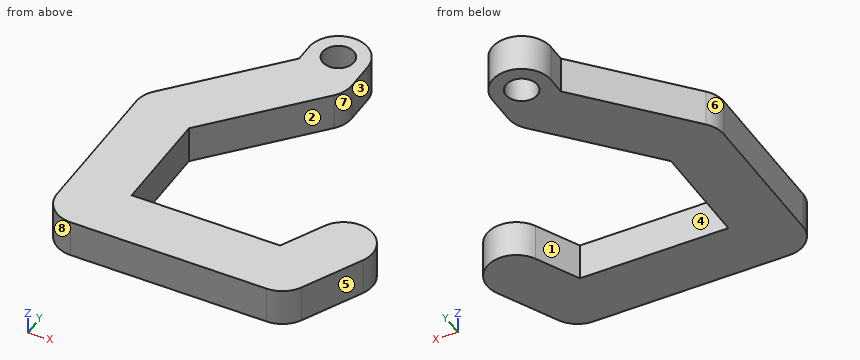
Autodesk Inventor part; units mm, degrees
ref_plane "YZ Plane" through (0, 0, 0) normal (1, 0, 0) x (0, 1, 0)
ref_plane "XZ Plane" through (0, 0, 0) normal (0, 1, 0) x (-1, 0, 0)
ref_plane "XY Plane" through (0, 0, 0) normal (0, 0, 1) x (1, 0, 0)
sketch "Sketch1" plane through (0, 0, 0) normal (0, 0, 1) x (1, 0, 0)
  circle A0 centre (0, 0) radius 1.6
  arc A1 (3, 0) -> (-3, 0) centre (0, 0) ccw
  line L0 (-3, 0) -> (-3, -1.8541)
  line L1 (-3, -3) -> (3, -3) construction
  line L2 (3, -3) -> (3, 0)
  arc A2 (-2.2361, -1) -> (-3, -3) centre (0, -3) ccw construction
  arc A3 (-13, -29.1803) -> (-10, -32.1803) centre (-10, -29.1803) ccw
  arc A4 (7, -29.1803) -> (12.6833, -30.522) centre (10, -29.1803) ccw
  arc A5 (15.6833, -24.522) -> (10.3167, -21.8387) centre (13, -23.1803) ccw
  arc A6 (-12.2361, -12.1803) -> (-13, -14.1803) centre (-10, -14.1803) ccw
  line L3 (-10, -29.1803) -> (10, -29.1803) construction
  line L4 (-7.7639, -16.1803) -> (-7, -15.3262)
  line L5 (-12.2361, -12.1803) -> (-3, -1.8541)
  line L6 (-13, -14.1803) -> (-13, -29.1803)
  line L7 (-7, -14.1803) -> (-7, -15.3262)
  line L8 (-10, -26.1803) -> (-7, -26.1803)
  line L9 (-10, -32.1803) -> (10, -32.1803)
  line L10 (10.3167, -21.8387) -> (7.3167, -27.8387)
  line L11 (12.6833, -30.522) -> (15.6833, -24.522)
  line L12 (-3, -1.8541) -> (-2.2361, -1) construction
  arc A7 (3, -3) -> (-2.2361, -1) centre (0, -3) ccw
  arc A8 (-3, -3) -> (2.2361, -5) centre (0, -3) ccw construction
  line L13 (-3, -1.8541) -> (-3, -3) construction
  arc A9 (2.2361, -5) -> (3, -3) centre (0, -3) ccw
  line L14 (-7, -15.3262) -> (2.2361, -5)
  line L15 (-7, -15.3262) -> (-7, -26.1803)
  arc A10 (-13, -14.1803) -> (-7, -14.1803) centre (-10, -14.1803) ccw construction
  line L16 (-7, -26.1803) -> (10, -26.1803)
  line L17 (-7, -26.1803) -> (-7, -29.1803)
  arc A11 (-10, -26.1803) -> (-13, -29.1803) centre (-10, -29.1803) ccw construction
  arc A12 (-10, -32.1803) -> (-10, -26.1803) centre (-10, -29.1803) ccw construction
  arc A13 (7.3167, -27.8387) -> (7, -29.1803) centre (10, -29.1803) ccw construction
  arc A14 (10, -26.1803) -> (7.3167, -27.8387) centre (10, -29.1803) ccw construction
  arc A15 (12.6833, -30.522) -> (10, -26.1803) centre (10, -29.1803) ccw construction
  arc A16 (10.3167, -21.8387) -> (15.6833, -24.522) centre (13, -23.1803) ccw construction
  point P0 (0, -29.1803)
  point P1 (8.1459, -26.1803)
  dimension "d0" = 3.2
  dimension "d1" = 6
  dimension "d2" = 3
  dimension "d3" = 6
  dimension "d4" = 6
  dimension "d5" = 6
  dimension "d6" = 6
  dimension "d7" = 15
  dimension "d8" = 6
  dimension "d9" = 15
  dimension "d10" = 20
  dimension "d11" = 3
  dimension "d12" = 6
extrude "Extrusion1" add sketch "Sketch1" along normal blind 3.8
properties part number "carlig 2"
Build history of the part. All positions in model axes, mm. Face numbers are marked on the shaded views. A direction names the side the tool comes from. Round coordinates to 2 decimals unless told otherwise and drop trailing zeros. Write each loop counter-clockwise with the first axis right and the second up, starting at its lowest first coordinate (ties: lowest second). Pieces come first, ordered by that corner, then holes. Notation, with made-up numbers: M -27,41.5 L 2,41.5 A18 cw 2,64.5 Z; hole C 73,53.25 d8. An arc over 180 degrees is marked long. Answer as a JSON object with one key per item and string values. Group by question number.
(1) Cut at A-A (z = 2.3). Give the cut face in (x, y).
(2) Cut at D-D (y = -17). Give the cut face in (x, z).
(3) Drill centre lines: L1, parallel to Y at x = 0, z = 1.2; L2, parallel to Y at x = -0.25, z = 2.1; L3, parallel to Y at x = 3.75, z = 2.85. Where is each one in solid material? Low to high.
(4) Flat gauge pins, fed straight in: pin 1 (2 mm diameter, centred on x = 0, y = -1, fed in from +Z); pin 2 (1.1 mm diameter, centred on y = -19.5, z = 1, fed in from +X); pin 3 (1.5 mm diameter, centred on y = -2, z = 1.5, fed in from +X); pin 4 (1.5 mm diameter, centred on y = -1, z = 1.5, fed in from -X). Where does each tip first touch, or does it go through?
(5) Mould opens along Y. For the marked faces 6, 7 and 8 say: pulls with the +Y half, pulls with the -Y half, needs draft (parallel to the pull), parting line crosses it, or undercut.
(6) Cut at C-C (y = -23.5). Give the cut face in (x, z), and give its area (3 significant figures).
(7) Cut at B-B (x = 0). Give the cut face in (y, z).
(8) Which spindle directions (+Z, -Z, +X, -X, +Y, -Y) get a long thin tool onto all of the face, cutting with end or side? Do the marked faces 1, 2, 3, 4 and 5. Say none if no direction does.
Responses:
{
 "1": {"outline": "M -13,-29.18 A3 ccw -10,-32.18 L 10,-32.18 A3 ccw 12.68,-30.52 L 15.68,-24.52 A3 ccw 10.32,-21.84 L 8.15,-26.18 L -7,-26.18 L -7,-15.33 L 2.24,-5 A3 ccw 3,-3 L 3,0 A3 ccw -3,0 L -3,-1.85 L -12.24,-12.18 A3 ccw -13,-14.18 Z; hole C 0,0 d3.2"},
 "2": {"outline": "M -13,0 L -7,0 L -7,3.8 L -13,3.8 Z"},
 "3": {"L1": "y = -32.18 to -26.18, -7.5 to -1.6, 1.6 to 3", "L2": "y = -32.18 to -26.18, -7.78 to -1.58, 1.58 to 2.99", "L3": "y = -32.18 to -26.18"},
 "4": {"pin 1": "stops at z = 3.8", "pin 2": "stops at x = -7", "pin 3": "stops at x = 3", "pin 4": "stops at x = -3"},
 "5": {"face 6": "pulls with the +Y half", "face 7": "undercut", "face 8": "pulls with the -Y half"},
 "6": {"outline": "M -13,0 L -7,0 L -7,3.8 L -13,3.8 Z; M 9.49,0 L 15.98,0 L 15.98,3.8 L 9.49,3.8 Z", "area": "47.5 mm2"},
 "7": {"outline": "M -32.18,0 L -26.18,0 L -26.18,3.8 L -32.18,3.8 Z; M -7.5,0 L -1.6,0 L -1.6,3.8 L -7.5,3.8 Z; M 1.6,0 L 3,0 L 3,3.8 L 1.6,3.8 Z"},
 "8": {"face 1": "+Z, -Z, +Y", "face 2": "+Z, -Z, +X", "face 3": "+Z, -Z, +X, +Y", "face 4": "+Z, -Z", "face 5": "+Z, -Z, +X, -Y"}
}
